Read the model definition and answer for the solid it produces. Units are mm, in the model's axes. A direction names the side the tool comes from. Coordinates: 2 decimals unless noted, no trailing zeros. Order: outer loops, then holes, each group sorted by start corner. A loop starts at its lowest first (then second) coordinate and runs counter-clockwise, first axis right, second up. Notation, with made-up numbers: (65.25, -37) -> (80.25, -37) arc R20 ccw to (80.25, -27) -> close; hole circle Ø8 at (-36.75, -39). An arc over 180 degrees is marked (long way). Use CSV: the item, a comma, the result in double quotes.
```python
from build123d import *


with BuildPart() as part:
    # Szkic1 → Obrót1 (revolve)
    with BuildSketch(Plane(origin=(0, 0, 0), x_dir=(0, 0, -1), z_dir=(1, 0, 0))):
        Polygon((-55, 0), (55, 0), (55, -7.5), (53.1, -7.5), (53.1, -7.15), (52, -7.15), (52, -7.5), (20, -7.5), (20, -9), (-20, -9), (-20, -7.5), (-52, -7.5), (-52, -7.15), (-53.1, -7.15), (-53.1, -7.5), (-55, -7.5), align=None)
    revolve(axis=Axis((0, 0, 55), (0, 0, -1)))


solid = part.part
```
Item 1: A tool of negligible diameter and unlimited length cuts with its end or side. For faces 4 (the cylindrical face through (-0.33, 7.493, 54.063)), 5 (the cylindrical face through (-0.33, 7.493, -54.037)), 6 (the cylindrical face through (-7.09, 0.93, -52.54)), from which of +Z, -Z, +X, -X, +Y, -Y can it reach the whole face along a straight path? Write none if from no direction.
Return value:
face 4,"+Z"
face 5,"-Z"
face 6,"none"
Item 2: Straight lines are drawn through the part: line 1 along Z through (x, y) = (-7, -2); line 2 along Z through (x, y) = (7.5, -3.75); line 3 along X through (y, z) = (0, 39). For each, find the intervals that lie inside material, in ascending order.
Return value:
line 1,"z = -55 to -53.1, -52 to 52, 53.1 to 55"
line 2,"z = -20 to 20"
line 3,"x = -7.5 to 7.5"
Item 3: Find section C-C, the plane z = 21.5. Give the vertices of the cut face in (x, y), then the cut area to 3 significant figures.
Return value:
outline,"circle Ø15 at (0, 0)"
area,"177 mm^2"
Item 4: Find section A-A, the plane x = 0. Give the vertices of the cut face in (y, z), then the cut area to 3 significant figures.
Return value:
outline,"(-9, -20) -> (-7.5, -20) -> (-7.5, -52) -> (-7.15, -52) -> (-7.15, -53.1) -> (-7.5, -53.1) -> (-7.5, -55) -> (7.5, -55) -> (7.5, -53.1) -> (7.15, -53.1) -> (7.15, -52) -> (7.5, -52) -> (7.5, -20) -> (9, -20) -> (9, 20) -> (7.5, 20) -> (7.5, 52) -> (7.15, 52) -> (7.15, 53.1) -> (7.5, 53.1) -> (7.5, 55) -> (-7.5, 55) -> (-7.5, 53.1) -> (-7.15, 53.1) -> (-7.15, 52) -> (-7.5, 52) -> (-7.5, 20) -> (-9, 20) -> close"
area,"1,770 mm^2"
Item 5: Find section D-D, the plane z = -12. Give the vertices of the cut face in (x, y), then the cut area to 3 significant figures.
Return value:
outline,"circle Ø18 at (0, 0)"
area,"254 mm^2"
Item 6: The mould has two halves that part along Z. Classify faces 1 (the flat face through (0, 0, 55)), 2 (the cylindrical face through (-7.09, 0.93, 52.56)), 3 (the flat face through (0, 0, -55)): +Z half, -Z half, draft (parallel to the pull), parting line (faces both ways), or undercut.
Return value:
face 1,"+Z half"
face 2,"undercut"
face 3,"-Z half"
Item 7: Each of these flat-tipped pins is pushed along its axis until it touches: P1, Ø2, axis at y = -5.5, z = -1.5, coming from the +X side; P2, Ø1.5, axis at x = 6.5, z = 24, coming from the +Y side; P3, Ø3, axis at x = -4.5, z = 33, coming from the -Y side. Where does it stop, or does it pass through?
Return value:
P1,"stops at x = 7.79"
P2,"stops at y = 4.82"
P3,"stops at y = -6.87"
